The listing builds one solid part. Answer for the finished solid, in the listing's coordinates (mm). Face numbers are marked on the shaded views. Give positions to 0.01 mm unless a question says otherwise; leave off trailing zeros. Order: outer loops, then holes, each group sorted by start corner. A loop starts at its lowest first (then second) coordinate and runs counter-clockwise, first axis right, second up. Notation, with made-up numbers: (38.5, 69) - (81.5, 69) arc R26 cw to (81.5, 93) - close; hole circle Ø2 at (-0.75, -25). An arc over 180 degrees is marked (long way). Use CSV: the item, a comma, the result in double quotes.
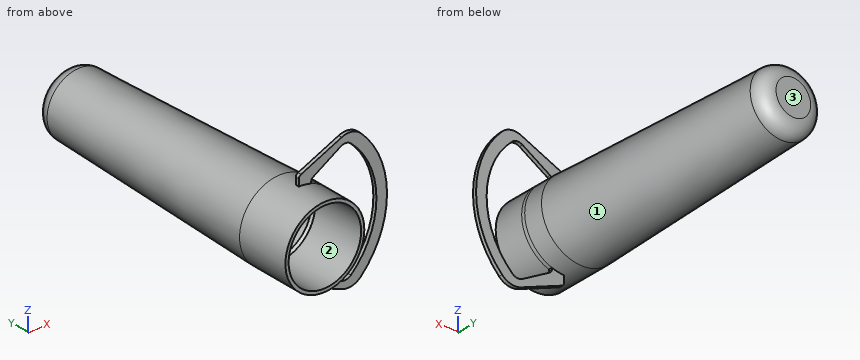
```python
from build123d import *

# Parameters (mm, degrees)
F2_R     = 20.575
F3_DEPTH = 2
F4_R     = 22.4
F4_R_2   = 20.575
F5_DEPTH = 17
F6_DEPTH = 30


# Not quite as in the source:
# - ends of sketch curves that miss each other by under 0.0002 mm in the source are joined


with BuildPart() as f3:
    # F2 (on Front) → F3 (new body)
    with BuildSketch(Plane.XZ):
        with BuildLine():
            Line((-13.8, 76.965483), (-13.8, 73.198817))
            ThreePointArc((-13.8, 73.198817), (-36.2, 50.798817), (-13.8, 28.398817))
            Line((-13.8, 28.398817), (-13.8, 24.63215))
            ThreePointArc((-13.8, 24.63215), (-13.464101, 23.52275), (-12.569231, 22.785996))
            Line((-12.569231, 22.785996), (10.519527, 13.16568))
            ThreePointArc((10.519527, 13.16568), (16.285797, 12.582523), (21.407101, 15.295858))
            ThreePointArc((21.407101, 15.295858), (36.2, 50.798817), (21.407101, 86.301775))
            ThreePointArc((21.407101, 86.301775), (16.285797, 89.01511), (10.519527, 88.431952))
            Line((10.519527, 88.431952), (-12.569231, 78.811637))
            ThreePointArc((-12.569231, 78.811637), (-13.464101, 78.074883), (-13.8, 76.965483))
        make_face()
        with Locations((-13.8, 50.798817)):
            Circle(F2_R, mode=Mode.SUBTRACT)
        with BuildLine():
            ThreePointArc((-6.8, 29.520659), (8.6, 50.798817), (-6.8, 72.076975))
            Line((-6.8, 72.076975), (-6.8, 73.151537))
            ThreePointArc((-6.8, 73.151537), (-6.534832, 74.146705), (-5.809641, 74.877986))
            Line((-5.809641, 74.877986), (9.844156, 84.032447))
            ThreePointArc((9.844156, 84.032447), (12.883236, 84.689734), (15.723162, 83.423698))
            ThreePointArc((15.723162, 83.423698), (30.2, 50.798817), (15.723162, 18.173935))
            ThreePointArc((15.723162, 18.173935), (12.883236, 16.907899), (9.844156, 17.565186))
            Line((9.844156, 17.565186), (-5.809641, 26.719647))
            ThreePointArc((-5.809641, 26.719647), (-6.534832, 27.450928), (-6.8, 28.446096))
            Line((-6.8, 28.446096), (-6.8, 29.520659))
        make_face(mode=Mode.SUBTRACT)
    extrude(amount=F3_DEPTH)

    # F4 (on face) → F5 (join)
    with BuildSketch(Plane.XZ.offset(2)):
        with Locations((-13.8, 50.798817)):
            Circle(F4_R)
        with Locations((-13.8, 50.798817)):
            Circle(F4_R_2, mode=Mode.SUBTRACT)
    extrude(amount=F5_DEPTH)

    # F6 (add): a face of the model
    f6_faces = [f3.faces().sort_by_distance(p)[0] for p in [
        (-35.566432, -19, 50.798817),
    ]]
    extrude(f6_faces, amount=-F6_DEPTH)

    # F7 (on plane+point) → F8 (revolve)
    with BuildSketch(Plane.XY.offset(50.798817)):
        with BuildLine():
            Line((6.7625, 11), (8.6, 11))
            Line((8.6, 11), (4.015629, 142.279196))
            ThreePointArc((4.015629, 142.279196), (1.57777, 147.754718), (-3.979497, 150))
            Line((-3.979497, 150), (-13.8, 150))
            Line((-13.8, 150), (-13.8, 148))
            Line((-13.8, 148), (-4.014418, 148))
            ThreePointArc((-4.014418, 148), (-0.541126, 146.596699), (0.982536, 143.174497))
            Line((0.982536, 143.174497), (5.556041, 12.206459))
            Line((5.556041, 12.206459), (6.7625, 11))
        make_face()
    revolve(axis=Axis((-13.8, 149, 50.798817), (0, -1, 0)))


solid = f3.part
```
Item 1: The part is cut by section B-B (y = 126.5). Give the vertices of the cut face in (x, z).
Taken from the geometry:
outline,"circle Ø36.73 at (-13.8, 50.8); hole circle Ø30.73 at (-13.8, 50.8)"
Item 2: Each of these flat-tipped pins is pushed along its axis until it touches: pin 1 (2 mm diameter, centred on y = -1, z = 26.5, fed in from -X); pin 2 (0.5 mm diameter, centred on y = -0.5, z = 29, fed in from +X); pin 3 (4 mm diameter, centred on y = 111.5, z = 48, fed in from +X). Where does it stop, or does it pass through?
Taken from the geometry:
pin 1,"x = -13.8"
pin 2,"x = 31.32"
pin 3,"x = 5.1"
Item 3: Find the intervals of material crossed by line 1 along Z through (x, y) = (-13, -4); line 2 along Z through (x, y) = (-5.5, 15.5); line 3 along X through (y, z) = (15, 61.5), in increasing order.
Taken from the geometry:
line 1,"28.41 to 30.24, 71.36 to 73.18"
line 2,"30.16 to 33.44, 68.16 to 71.44"
line 3,"-33.32 to -29.81, 2.21 to 5.72"
Item 4: The mould has two halves that part along Z. Classify the marked faces 1, 2 and 3: +Z half, -Z half, draft (parallel to the pull), parting line (faces both ways), or undercut.
Taken from the geometry:
face 1,"parting line"
face 2,"undercut"
face 3,"draft"
Item 5: The part is cut by section C-C (y = 95.5). Give the vertices of the cut face in (x, z).
Taken from the geometry:
outline,"circle Ø38.9 at (-13.8, 50.8); hole circle Ø32.89 at (-13.8, 50.8)"
Item 6: The part is cut by section A-A (x = 13). Give the vertices of the cut face in (y, z), and give its area (3 significant figures).
Taken from the geometry:
outline,"(-2, 12.49) - (0, 12.49) - (0, 16.92) - (-2, 16.92) - close; (-2, 84.68) - (0, 84.68) - (0, 89.11) - (-2, 89.11) - close"
area,"17.7 mm^2"
